Part model, mm, in its own coordinate system. A direction names the side the tool comes from. Coordinates: 2 decimals unless noted, no trailing zeros. Loops run counter-clockwise (first coordinate to the right, second up) from the corner with the lowest first, then second, coordinate; pieces in that order, holes last. Notation, with made-up numbers: (19.5, -38) - (40.5, -38) arc R17 cw to (40.5, -30) - close; hole circle Ø9 at (50, 87). An arc over 180 degrees is marked (long way). Use a Markdown table: item, result. Add a question column.
1) Probe probe 1 along X at (y, z) = (-238.5, -6); probe 2 along Y at (x, z) = (-61, 6.5); probe 3 along Z at (x, y) = (26, -37.5). List the from-to ranges inside material, lowest first. Write a range as [from, to].
2) Band-saw the part on C-C (y = -186.5). Give the cut face in (x, z), plus the area to 3 significant figures.
3) Band-saw the part on A-A (z = 1). Give the cut face in (x, y), plus the area to 3 significant figures.
4) Tool access for faces 1 (the face through (43.717, -125, 15)), 2 (the face through (-71.898, -125, 16)): list every direction of +Z, -Z, +X, -X, +Y, -Y with a clear straight run to the whole face (end or side of a thin tool).
5) Pull direction Z, two halves, no side cores. Call faces 3 (the face through (-60, -32, -37.787)), 4 (the face through (-16, -247.65, 18)), 5 (the face through (14.166, -125.222, 98.287)), 6 (the face through (-17, -125, -44.137)): +Z half, -Z half, draft (parallel to the pull), parting line (faces both ways), or undercut.
6) Band-saw the part on B-B (x = 3). Give the cut face in (y, z).
7) Band-saw the part on D-D (z = 43.5). Give the cut face in (x, y), plus the area to 3 significant figures.
8) Drop flat-ended pins along their axis: P1, Ø1, axis at x = 11, y = -75, coming from the +Z side; P2, Ø4, axis at x = 2, y = -76, coming from the +Z side; P3, Ø9.5, axis at x = -60, y = -23, coming from the +Z side. Give the stop position or say it passes through.
from build123d import *

# Parameters (mm, degrees)
F0_W     = 119.885028
F0_H     = 119.885028
F1_DEPTH = 254
F2_W     = 109.586086
F2_H     = 111.699324
F3_DEPTH = 247.65
F4_W     = 31.353211
F4_H     = 60.86609
F5_DEPTH = 25.4
F6_W     = 116.465766
F6_H     = 116.456397
F7_DEPTH = 6.35
F8_W     = 32.10051
F8_H     = 42.383331
F9_DEPTH = 6.35


with BuildPart() as f1:
    # F0 (on Front) → F1 (new body)
    with BuildSketch(Plane.XZ):
        Polygon((-16.225174, 121.46537), (-76.167688, 75.748228), (43.71734, 75.748228), align=None)
        with Locations((-16.225174, 15.805714)):
            Rectangle(F0_W, F0_H)
    extrude(amount=F1_DEPTH)

    # F2 (on face) → F3 (cut)
    with BuildSketch(Plane(origin=(0, 0, 0), x_dir=(-1, 0, 0), z_dir=(0, 1, 0))):
        with Locations((17.105127, 17.154949)):
            Rectangle(F2_W, F2_H)
    extrude(amount=-F3_DEPTH, mode=Mode.SUBTRACT)

    # F4 (on face) → F5 (cut)
    with BuildSketch(Plane(origin=(-76.167688, 0, 0), x_dir=(0, -1, 0), z_dir=(-1, 0, 0))):
        with Locations((30.565259, -13.703755)):
            Rectangle(F4_W, F4_H)
    extrude(amount=-F5_DEPTH, mode=Mode.SUBTRACT)

    # F6 (on Front) → F7 (join)
    with BuildSketch(Plane.XZ):
        with Locations((-15.793322, 16.630638)):
            Rectangle(F6_W, F6_H)
    extrude(amount=F7_DEPTH)

    # F8 (on face) → F9 (join)
    with BuildSketch(Plane(origin=(0, 0, -44.1368), x_dir=(1, 0, 0), z_dir=(0, 0, -1))):
        with Locations((-60.117433, 31.530009)):
            Rectangle(F8_W, F8_H)
    extrude(amount=-F9_DEPTH)


solid = f1.part
Answer block:
| question | item | result |
|---|---|---|
| 1 | probe 1 | [-76.17, -71.9], [37.69, 43.72] |
| 1 | probe 2 | [-254, -247.65], [-6.35, 0] |
| 1 | probe 3 | [-44.14, -38.69], [73, 89.26] |
| 2 | outline | (-76.17, -44.14) - (43.72, -44.14) - (43.72, 75.75) - (-16.23, 121.47) - (-76.17, 75.75) - close; hole (-71.9, -38.69) - (37.69, -38.69) - (37.69, 73) - (-71.9, 73) - close |
| 2 | area | 4,870 mm2 |
| 3 | outline | (-76.17, -254) - (43.72, -254) - (43.72, 0) - (-76.17, 0) - (-76.17, -14.89) - (-71.9, -14.89) - (-71.9, -6.35) - (37.69, -6.35) - (37.69, -247.65) - (-71.9, -247.65) - (-71.9, -46.24) - (-76.17, -46.24) - close |
| 3 | area | 3,870 mm2 |
| 4 | face 1 | +Z, -Z, +X, +Y, -Y |
| 4 | face 2 | none |
| 5 | face 3 | undercut |
| 5 | face 4 | undercut |
| 5 | face 5 | +Z half |
| 5 | face 6 | -Z half |
| 6 | outline | (-254, -44.14) - (0, -44.14) - (0, 106.8) - (-254, 106.8) - close; hole (-247.65, -38.69) - (-6.35, -38.69) - (-6.35, 73) - (-247.65, 73) - close |
| 7 | outline | (-76.17, -254) - (43.72, -254) - (43.72, 0) - (-76.17, 0) - close; hole (-71.9, -247.65) - (37.69, -247.65) - (37.69, -6.35) - (-71.9, -6.35) - close |
| 7 | area | 4,010 mm2 |
| 8 | P1 | z = 101.08 |
| 8 | P2 | z = 109.09 |
| 8 | P3 | z = 91.7 |
